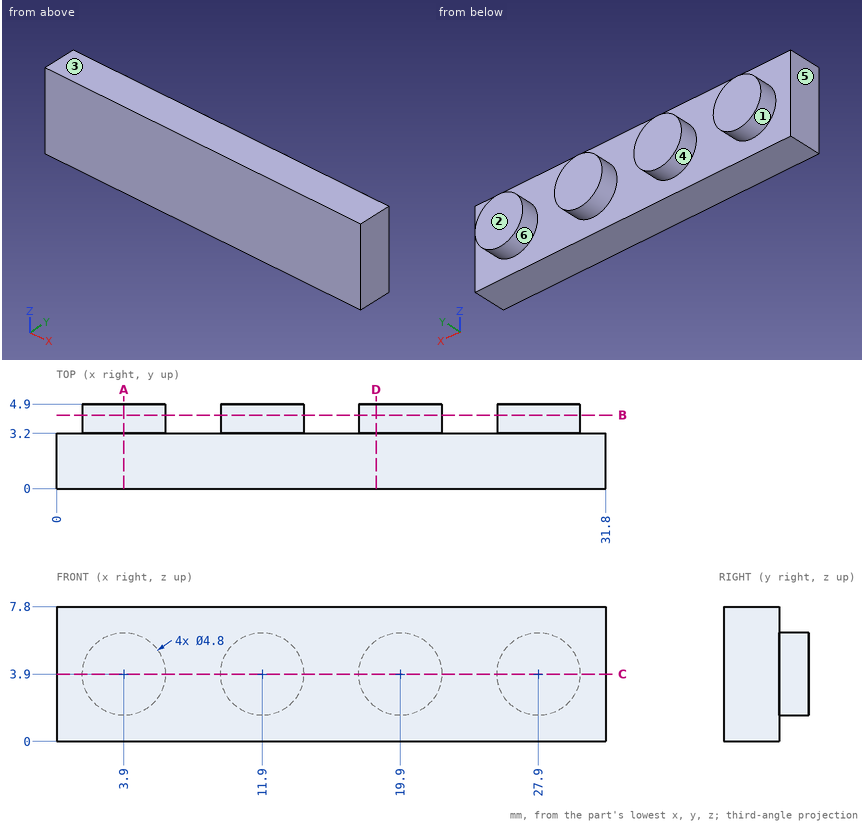
Print and shaded views of the part. All mm, measured from the part's lowest x, y and z. A direction names the side the tool comes from. Round coordinates to 2 decimals unless told otherwise and drop trailing zeros. Write each loop counter-clockwise with the first axis right and the second up, starting at its lowest first coordinate (ties: lowest second). Pieces come first, ordered by that corner, then holes.
(1) Slice it at D-D, the plane x = 18.5. Write the cut outline in (y, z).
(2) Mould opens along X. For the marked faces 3, 4, 5 and 6 say: pulls with the +X half, pulls with the -X half, needs draft (parallel to the pull), parting line crosses it, or undercut.
(3) Slice it at C-C, the plane z = 3.9. Write the cut outline in (x, y), and give its area (3 significant figures).
(4) Drop a flat-ended pin along its axis: P1, Ø1.5, axis at y = 4, z = 4.5, coming from the +X side. Give the stop position or say it passes through.
(5) Slice it at A-A, the plane x = 3.9. Write the cut outline in (y, z).
(6) 3-axis set-ups, long thin cutter, end or side, ignore diameter. For the marked faces 1 and 2: which of +Z, -Z, +X, -X, +Y, -Y reach the whole face in a straight line?
(7) Slice it at B-B, the plane y = 4.25. Write the cut outline in (x, z), and give its area (3 significant figures).
(8) Probe line 1 along X through (y, z) = (4.6, 4); line 2 along X through (y, z) = (4, 6); line 3 along Y through (x, z) = (24, 2.5). List the from-to ranges inside material, lowest first.
From the geometry:
1. outline: (0, 0) - (3.2, 0) - (3.2, 1.95) - (4.9, 1.95) - (4.9, 5.85) - (3.2, 5.85) - (3.2, 7.8) - (0, 7.8) - close
2. face 3: needs draft
2. face 4: undercut
2. face 5: pulls with the -X half
2. face 6: undercut
3. outline: (0, 0) - (31.8, 0) - (31.8, 3.2) - (30.3, 3.2) - (30.3, 4.9) - (25.5, 4.9) - (25.5, 3.2) - (22.3, 3.2) - (22.3, 4.9) - (17.5, 4.9) - (17.5, 3.2) - (14.3, 3.2) - (14.3, 4.9) - (9.5, 4.9) - (9.5, 3.2) - (6.3, 3.2) - (6.3, 4.9) - (1.5, 4.9) - (1.5, 3.2) - (0, 3.2) - close
3. area: 134 mm2
4. P1: stops at x = 30.3
5. outline: (0, 0) - (3.2, 0) - (3.2, 1.5) - (4.9, 1.5) - (4.9, 6.3) - (3.2, 6.3) - (3.2, 7.8) - (0, 7.8) - close
6. face 1: +Y
6. face 2: +Z, -Z, +X, -X, +Y
7. outline: circle Ø4.8 at (3.9, 3.9); circle Ø4.8 at (11.9, 3.9); circle Ø4.8 at (19.9, 3.9); circle Ø4.8 at (27.9, 3.9)
7. area: 72.4 mm2
8. line 1: x = 1.5 to 6.3, 9.5 to 14.3, 17.5 to 22.3, 25.5 to 30.3
8. line 2: x = 2.74 to 5.06, 10.74 to 13.06, 18.74 to 21.06, 26.74 to 29.06
8. line 3: y = 0 to 3.2
